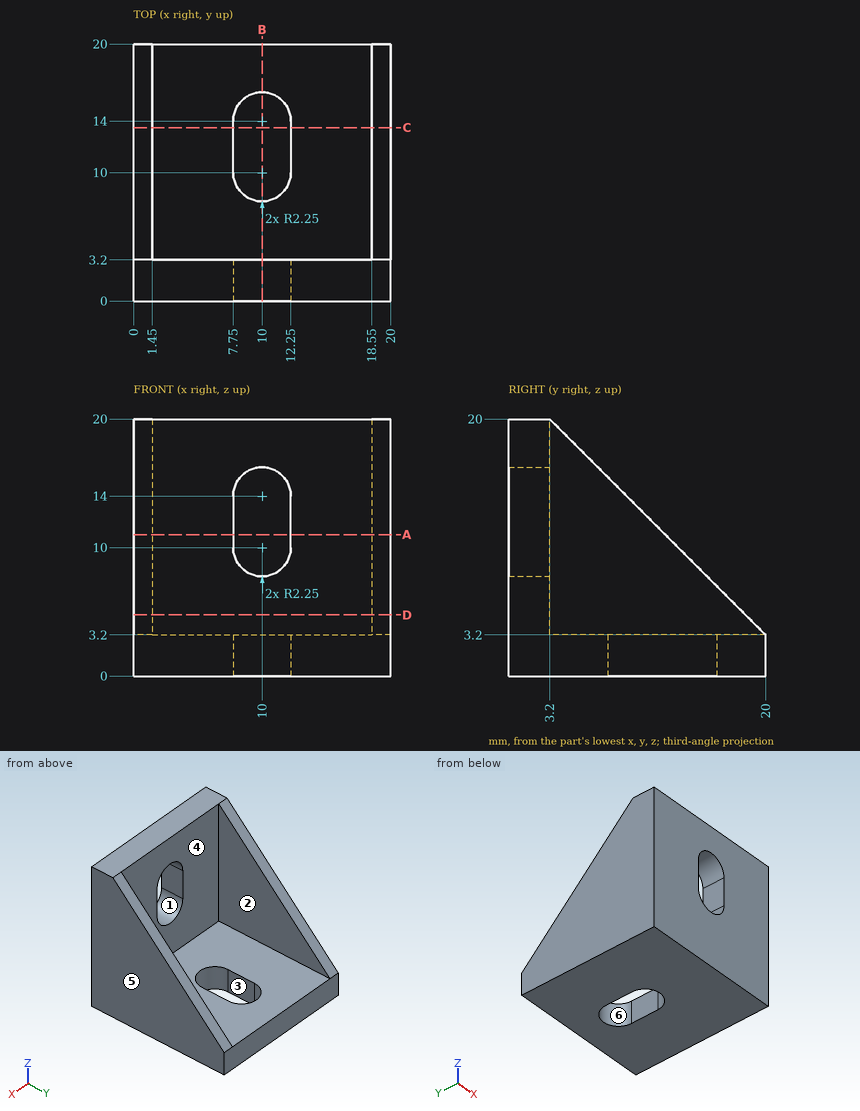
Source: three-view drawing plus pictorial views. Frame: mm from the lowest corner of the part. A direction names the side the tool comes from. Coordinates: 2 decimals unless noted, no trailing zeros. Loops run counter-clockwise (first coordinate to the right, second up) from the corner with the lowest first, then second, coordinate; pieces in that order, holes last. Notation, with made-up numbers: (1, 5.5) -> (28, 5.5) arc R19 ccw to (28, 20.5) -> close; hole circle Ø11 at (40.5, 45). An arc over 180 degrees is marked (long way). Write each question's results on one line, items separated by ' | '. Start each with the question number.
Q1. Reachability of the marked faces 1, 2 and 3 from +Z, -Z, +X, -X, +Y, -Y: full face, straight path, thin tool, end or side. Return the list, or none.
Q2. Section B-B, the plane x = 10. Return the cut outline in (y, z), plus the area to 3 significant figures.
Q3. Ray query, line 1 (X direction, y = 3.25, z = 12); line 2 (Y direction, x = 7, z = 6.25). Return the intervals inside material, ascending. Write a range as from..to.
Q4. Pin query (flat end, axial travel): pin 1 (12 mm diameter, centred on y = 12, z = 13, fed in from -X); pin 2 (5 mm diameter, centred on x = 6, y = 12.5, fed in from +Z); pin 3 (6 mm diameter, centred on x = 4.5, z = 12.5, fed in from +Y). Return the tip coordinate at first contact, or that it passes through.
Q5. Pull-direction query (Y, two-part tool) for the marked faces 4, 5 and 6; classes: released by +Y, released by -Y, zero draft, split by the parting line, or undercut.
Q6. Section D-D, the plane z = 4.75. Return the cut outline in (x, y), plus the area to 3 significant figures.
Q7. Section C-C, the plane y = 13.5. Return the cut outline in (x, z).
Q8. Section A-A, the plane z = 11. Return the cut outline in (x, y), plus the area to 3 significant figures.
Found:
1) face 1: +Y, -Y | face 2: +Z, +Y | face 3: +Z, -Z
2) outline: (0, 0) -> (7.75, 0) -> (7.75, 3.2) -> (3.2, 3.2) -> (3.2, 7.75) -> (0, 7.75) -> close; (0, 16.25) -> (3.2, 16.25) -> (3.2, 20) -> (0, 20) -> close; (16.25, 0) -> (20, 0) -> (20, 3.2) -> (16.25, 3.2) -> close | area: 63.4 mm2
3) line 1: 0..1.45, 18.55..20 | line 2: 0..3.2
4) pin 1: x = 0 | pin 2: z = 3.2 | pin 3: y = 3.2
5) face 4: released by +Y | face 5: zero draft | face 6: undercut
6) outline: (0, 0) -> (20, 0) -> (20, 18.45) -> (18.55, 18.45) -> (18.55, 3.2) -> (1.45, 3.2) -> (1.45, 18.45) -> (0, 18.45) -> close | area: 108 mm2
7) outline: (0, 0) -> (7.75, 0) -> (7.75, 3.2) -> (1.45, 3.2) -> (1.45, 9.7) -> (0, 9.7) -> close; (12.25, 0) -> (20, 0) -> (20, 9.7) -> (18.55, 9.7) -> (18.55, 3.2) -> (12.25, 3.2) -> close
8) outline: (0, 0) -> (7.75, 0) -> (7.75, 3.2) -> (1.45, 3.2) -> (1.45, 12.2) -> (0, 12.2) -> close; (12.25, 0) -> (20, 0) -> (20, 12.2) -> (18.55, 12.2) -> (18.55, 3.2) -> (12.25, 3.2) -> close | area: 75.7 mm2
